Check sheet for the modelled part. Datum: model origin and axes. Units: mm. Face numbers are marked on the shaded views. A direction names the side the tool comes from. Give positions to 0.01 mm unless a question says otherwise; leave off trailing zeros. Write each loop counter-clockwise with the first axis right and the second up, starting at its lowest first coordinate (ties: lowest second). Pieces come first, ordered by that corner, then holes. Notation, with made-up numbers: (-10.5, -36) -> (28.5, -36) arc R6 cw to (28.5, -31) -> close; hole circle Ø8 at (78.5, 41). An arc over 180 degrees is marked (long way). Use a Markdown table: item, result. Add a question column.
1. Cross-section at A-A (z = -4.5). Enter the section's corners in (x, y) (1 decimal), then the cut area to 3 significant figures.
2. Set-up check for the marked faces 4, 5 and 6: record each of +Z, -Z, +X, -X, +Y, -Y from which the full face is reachable in a straight line by a thin tool's end or side.
3. Release check for a two-part mould opening along Z. For the marked faces 1, 2 and 3 record: released by +Z, released by -Z, zero draft, split by the parting line, or undercut.
4. Gauge pin test, flat ends, axial feed: P1, Ø1.5, axis at x = 5, z = 2.5, coming from the +Y side; P2, Ø1, axis at x = 6.5, z = 16.5, coming from the -Y side (3 decimals); P3, Ø4, axis at x = 8.5, y = 8.5, coming from the -Z side; P4, Ø5, axis at y = -11, z = 1, coming from the +X side. Record the tip position at first contact, or that the pin passes through.
5. Scan lines: probe 1 along Z at (x, y) = (10.25, -11); probe 2 along Y at (x, z) = (13, 1.5). Record each from-to range of solid material in increasing order. Write a range as [from, to].
6. Cross-section at D-D (y = -15). Enter the section's corners in (x, z) (3 decimals).
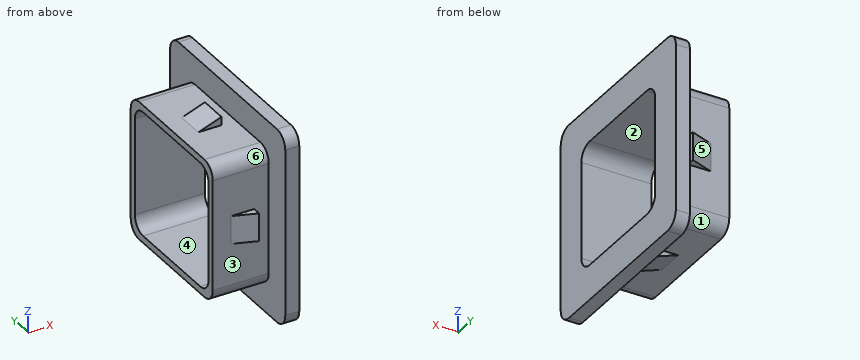
Autodesk Inventor part; units mm, degrees
ref_plane "YZ Plane" through (0, 0, 0) normal (1, 0, 0) x (0, 1, 0)
ref_plane "XZ Plane" through (0, 0, 0) normal (0, 1, 0) x (-1, 0, 0)
ref_plane "XY Plane" through (0, 0, 0) normal (0, 0, 1) x (1, 0, 0)
sketch "Sketch1" plane through (0, 0, 0) normal (1, 0, 0) x (0, 1, 0)
  line L0 (-15.748, -15.748) -> (15.748, -15.748)
  line L1 (15.748, -15.748) -> (15.748, 15.748)
  line L2 (15.748, 15.748) -> (-15.748, 15.748)
  line L3 (-15.748, 15.748) -> (-15.748, -15.748)
  line L4 (-15.748, -15.748) -> (15.748, 15.748) construction
  line L5 (15.748, -15.748) -> (-15.748, 15.748) construction
  line L6 (14.1605, 14.1605) -> (14.1605, -14.1605)
  line L7 (14.1605, -14.1605) -> (-14.1605, -14.1605)
  line L8 (-14.1605, -14.1605) -> (-14.1605, 14.1605)
  line L9 (-14.1605, 14.1605) -> (14.1605, 14.1605)
  point P0 (0, 0)
  dimension "d0" = 31.496
  dimension "d1" = 31.496
  dimension "d2" = 1.5875
extrude "Extrusion1" add sketch "Sketch1" along normal blind 12.7
sketch "Sketch2" plane through (12.7, 0, 0) normal (1, 0, 0) x (0, 0, -1)
  line L0 (15.748, 15.748) -> (-15.748, 15.748)
  line L1 (-15.748, 15.748) -> (-15.748, -15.748)
  line L2 (-15.748, -15.748) -> (15.748, -15.748)
  line L3 (15.748, -15.748) -> (15.748, 15.748)
  line L4 (-14.1605, 14.1605) -> (14.1605, 14.1605)
  line L5 (14.1605, 14.1605) -> (14.1605, -14.1605)
  line L6 (14.1605, -14.1605) -> (-14.1605, -14.1605)
  line L7 (-14.1605, -14.1605) -> (-14.1605, 14.1605)
  line L8 (-22.098, 22.098) -> (22.098, 22.098)
  line L9 (22.098, 22.098) -> (22.098, -22.098)
  line L10 (22.098, -22.098) -> (-22.098, -22.098)
  line L11 (-22.098, -22.098) -> (-22.098, 22.098)
  point P0 (0, 0)
  dimension "d5" = 6.35
extrude "Extrusion2" add sketch "Sketch2" along normal blind 3.175 contours L3 L2 L1 L0 | L8 L9 L10 L11
fillet "Fillet1" radius 3.175 12 edges at (6.35, 15.748, 15.748) (6.35, 15.748, -15.748) (6.35, -15.748, 15.748) (6.35, -15.748, -15.748) (7.9375, 14.1605, 14.1605) (7.9375, -14.1605, 14.1605) (7.9375, -14.1605, -14.1605) (7.9375, 14.1605, -14.1605) (14.2875, -22.098, 22.098) (14.2875, -22.098, -22.098) (14.2875, 22.098, -22.098) (14.2875, 22.098, 22.098)
sketch "Sketch4" plane through (0, 0, 0) normal (0, 0, 1) x (1, 0, 0)
  line L0 (0, -15.748) -> (12.7, -15.748) construction
  line L1 (4.1641, -15.748) -> (9.398, -17.653)
  line L2 (9.398, -17.653) -> (9.398, -15.748)
  line L3 (12.7, -18.923) -> (12.7, 18.923) construction
  line L4 (4.1641, -15.748) -> (9.398, -15.748)
  point P0 (0, 0)
  dimension "d9" = 3.302
  dimension "d10" = 1.905
  dimension "d11" = 20
extrude "Extrusion3" add sketch "Sketch4" along normal mid plane 6.35
pattern_circular "Circular Pattern1" count 4 over 360 about axis through (-10, 0, 0) along (1, 0, 0) of "Extrusion3"
properties part number "DB1-013" material "ABS Plastic"
Worked answers:
| question | item | result |
|---|---|---|
| 1 | outline | (0, -15.7) -> (12.7, -15.7) -> (12.7, -22.1) -> (15.9, -22.1) -> (15.9, -14.2) -> (0, -14.2) -> close; (0, 14.2) -> (15.9, 14.2) -> (15.9, 22.1) -> (12.7, 22.1) -> (12.7, 15.7) -> (0, 15.7) -> close |
| 1 | area | 90.7 mm² |
| 2 | face 4 | +X, -X |
| 2 | face 5 | +Z, -Z, -X, +Y |
| 2 | face 6 | +Z, -X, -Y |
| 3 | face 1 | released by -Z |
| 3 | face 2 | undercut |
| 3 | face 3 | zero draft |
| 4 | P1 | stops at y = 16.33 |
| 4 | P2 | stops at y = -3.175 |
| 4 | P3 | stops at z = -15.75 |
| 4 | P4 | passes through |
| 5 | probe 1 | z = [-15.75, -14.16], [14.16, 15.75] |
| 5 | probe 2 | y = [-22.1, -14.16], [14.16, 22.1] |
| 6 | outline | (0, -14.62) -> (12.7, -14.62) -> (12.7, -22.098) -> (15.875, -22.098) -> (15.875, 22.098) -> (12.7, 22.098) -> (12.7, 14.62) -> (0, 14.62) -> close |
